from build123d import *


with BuildPart() as part:
    # Sketch1 → Revolve1 (revolve)
    with BuildSketch(Plane(origin=(0, 0, 0), x_dir=(1, 0, 0), z_dir=(0, 1, 0))):
        with BuildLine():
            Line((0, 0), (5.4, 0))
            ThreePointArc((5.4, 0), (6.107106781, 0.292893219), (6.4, 1))
            Line((6.4, 1), (6.4, 5))
            Line((6.4, 5), (8, 5))
            Line((8, 5), (8, 9))
            Line((8, 9), (2.828427125, 9))
            ThreePointArc((2.828427125, 9), (1.732050808, 10.449489743), (0, 11))
            Line((0, 11), (0, 0))
        make_face()
    revolve(axis=Axis((0, 0, 0), (0, 0, -1)))


solid = part.part
Can you work these out from the model? Positions are in its coordinate system, mm. A direction names the side the tool comes from. Coordinates: 2 decimals unless noted, no trailing zeros. Write each loop counter-clockwise with the first axis right and the second up, starting at its lowest first coordinate (ties: lowest second). Pieces come first, ordered by that corner, then holes.
Q1. Please list where these lines run through material, in increasing order: L1, parallel to Z at x = 0, y = 4.5; L2, parallel to Z at x = -4, y = 4.25; L3, parallel to X at y = -1.5, z = -10.
Results found:
L1: z = -9 to 0
L2: z = -9 to -0.1
L3: x = -1.66 to 1.66
Q2. Imagine slicing it at D-D, the plane x = 6.75. List the corners of the cut face in (y, z) for me.
Results found:
outline: (-4.29, -9) - (4.29, -9) - (4.29, -5) - (-4.29, -5) - close
Q3. If we mould it in two halves opening along X, with no side actions, what happens to faces 1 (the face through (0, -7, -5)), 2 (the face through (-5.08, 3.89, -3.03))? For each: +X half, -X half, draft (parallel to the pull), parting line (faces both ways), or undercut.
Results found:
face 1: draft
face 2: parting line
Q4. Imagine slicing it at A-A, the plane x = 0. List the corners of the cut face in (y, z) for me.
Results found:
outline: (-8, -9) - (-2.83, -9) arc R3 ccw to (2.83, -9) - (8, -9) - (8, -5) - (6.4, -5) - (6.4, -1) arc R1 ccw to (5.4, 0) - (-5.4, 0) arc R1 ccw to (-6.4, -1) - (-6.4, -5) - (-8, -5) - close
Q5. Imagine slicing it at C-C, the plane z = -7.5. List the corners of the cut face in (x, y) for me.
Results found:
outline: circle Ø16 at (0, 0)
Q6. Which directions (+Z, -Z, +X, -X, +Y, -Y) give clear straight access to the entire face, cutting with the end or side of a thin tool? Please do faces 3 (the face through (0, 0, 0)), 4 (the face through (3, 0, -9)).
Results found:
face 3: +Z, +X, -X, +Y, -Y
face 4: -Z
Q7. For P1, Ø5, axis at x = -2.5, y = -1.5, coming from the -Z side; P2, Ø4, axis at y = -4.5, z = -5.5, coming from the +X side; P3, Ø2, axis at x = 0.5, z = -3, coming from the -Y side, each with a flat end and sliding along its axis, tell me the tip position at first contact or that it passes through.
Results found:
P1: stops at z = -10.97
P2: stops at x = 7.6
P3: stops at y = -6.4
